CAD build for the part. Positions are in the model's coordinates, mm. Face numbers are marked on the shaded views. A direction names the side the tool comes from. Round coordinates to 2 decimals unless told otherwise and drop trailing zeros. Write each loop counter-clockwise with the first axis right and the second up, starting at its lowest first coordinate (ties: lowest second). Pieces come first, ordered by that corner, then holes. Notation, with made-up numbers: (23.5, 89.25) - (67.5, 89.25) arc R5 ccw to (67.5, 94.25) - close; hole circle Ø1 at (-30.75, 89.25). An arc over 180 degrees is marked (long way). Put each result on its own line as item: value. Start each with the question number.
Item 1: Pin check, flat tips, straight feed: pin 1 Ø1 at (y, z) = (18, 11) entering from -X; pin 2 Ø1.4 at (x, z) = (-10, 11) entering from +Y; pin 3 Ø0.8 at (x, y) = (8.5, 20.5) entering from +Z. Stop position of each tip, or through.
Item 2: Cut at A-A (y = 15). Give the cut face in (x, z), and give its area (3 significant figures).
Item 3: 3-axis set-ups, long thin cutter, end or side, ignore diameter. For the marked faces 1, 2, 3, 4 and 5: which of +Z, -Z, +X, -X, +Y, -Y reach the whole face in a straight line?
Item 4: Cut at B-B (x = -24). Give the cut face in (y, z).
Item 5: Drill centre lines: line 1 (Y direction, x = -3, z = 5.5); line 2 (X direction, y = -13, z = 1.75); line 3 (Y direction, x = 22, z = 13). Where is each one in solid material? Low to high. Write a range as from..to.
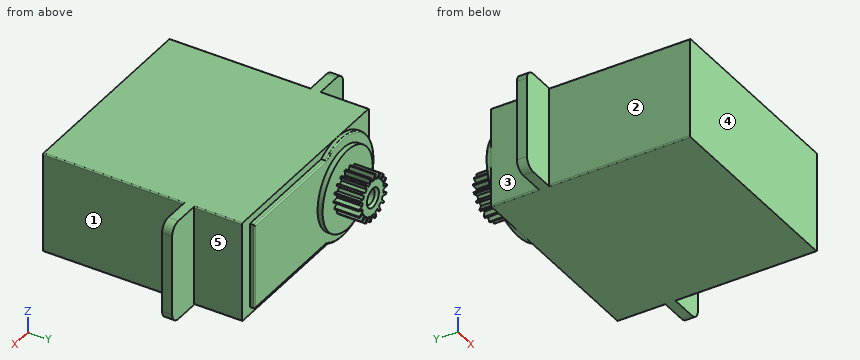
```python
from build123d import *

# Parameters (mm, degrees)
ESQUISSE1_W                  = 40.5
ESQUISSE1_H                  = 39.5
BOSS_EXTRU_1_DEPTH           = 20
ESQUISSE2_W                  = 20
ESQUISSE2_H                  = 2
BOSS_EXTRU_2_DEPTH           = 7
ESQUISSE3_W                  = 20
ESQUISSE3_H                  = 2
BOSS_EXTRU_3_DEPTH           = 7
CONG_1_R                     = 2
BOSS_EXTRU_4_DEPTH           = 1
ESQUISSE6_R                  = 8
BOSS_EXTRU_5_DEPTH           = 1
ESQUISSE7_R                  = 4.5
BOSS_EXTRU_6_DEPTH           = 5
ENL_V_START                  = -5
ENL_V_MAT_EXTRU_2_DEPTH      = 5
R_P_TITION_CIRCULAIRE2_COUNT = 18
ESQUISSE9_R                  = 1.4
ENL_V_MAT_EXTRU_3_DEPTH      = 5
CHANFREIN1_SIZE              = 0.5
CONG_3_R                     = 0.25
CONG_4_R                     = 0.25


with BuildPart() as part:
    # Esquisse1 → Boss.-Extru.1 (new body)
    with BuildSketch(Plane.XY):
        Rectangle(ESQUISSE1_W, ESQUISSE1_H)
    extrude(amount=BOSS_EXTRU_1_DEPTH)

    # Esquisse2 → Boss.-Extru.2 (add)
    with BuildSketch(Plane.ZY.offset(20.25)):
        with Locations((10, 9.25)):
            Rectangle(ESQUISSE2_W, ESQUISSE2_H)
    extrude(amount=BOSS_EXTRU_2_DEPTH)

    # Esquisse3 → Boss.-Extru.3 (add)
    with BuildSketch(Plane(origin=(20.25, 0, 0), x_dir=(0, 0, -1), z_dir=(1, 0, 0))):
        with Locations((-10, 9.25)):
            Rectangle(ESQUISSE3_W, ESQUISSE3_H)
    extrude(amount=BOSS_EXTRU_3_DEPTH)

    # Congé1
    cong_1_edges = [part.edges().sort_by_distance(p)[0] for p in [
        (-27.25, 9.25, 0),
        (-27.25, 9.25, 20),
        (27.25, 9.25, 20),
        (27.25, 9.25, 0),
    ]]
    fillet(cong_1_edges, radius=CONG_1_R)

    # Esquisse4 → Boss.-Extru.4 (add)
    with BuildSketch(Plane(origin=(0, 19.75, 0), x_dir=(1, 0, 0), z_dir=(0, 1, 0))):
        with BuildLine():
            Line((17.75, -1.5), (17.75, -18.5))
            Line((17.75, -18.5), (-5.001587186, -18.5))
            ThreePointArc((-5.001587186, -18.5), (-20.239786638, -10), (-5.001587186, -1.5))
            Line((-5.001587186, -1.5), (17.75, -1.5))
        make_face()
    extrude(amount=BOSS_EXTRU_4_DEPTH)

    # Esquisse6 → Boss.-Extru.5 (add)
    with BuildSketch(Plane(origin=(0, 20.75, 0), x_dir=(1, 0, 0), z_dir=(0, 1, 0))):
        with Locations(Location((-10.25, -10, 0), (0, 0, 270))):
            Circle(ESQUISSE6_R)
    extrude(amount=BOSS_EXTRU_5_DEPTH)

    # Esquisse7 → Boss.-Extru.6 (add)
    with BuildSketch(Plane(origin=(0, 21.75, 0), x_dir=(1, 0, 0), z_dir=(0, 1, 0))):
        with Locations(Location((-10.25, -10, 0), (0, 0, 270))):
            Circle(ESQUISSE7_R)
    extrude(amount=BOSS_EXTRU_6_DEPTH)

    # Esquisse8 → Enlèv. mat.-Extru.2 (cut)
    with BuildSketch(Plane(origin=(0, 26.75, 0), x_dir=(1, 0, 0), z_dir=(0, 1, 0)).offset(ENL_V_START)):
        with BuildLine():
            Line((-10.606352849, -6.656584169), (-10.903477232, -5.547700874))
            ThreePointArc((-10.903477232, -5.547700874), (-10.272597671, -5.50005674), (-9.641271425, -5.541362369))
            Line((-9.641271425, -5.541362369), (-9.940094206, -6.656584169))
            Line((-9.940094206, -6.656584169), (-10.606352849, -6.656584169))
        make_face()
    enl_v_mat_extru_2 = extrude(amount=ENL_V_MAT_EXTRU_2_DEPTH, mode=Mode.SUBTRACT)

    # Répétition circulaire2: Enlèv. mat.-Extru.2 ×18 about axis
    r_p_tition_circulaire2_axis = Axis((-10.249601616, 0, 10.07055578), (0, 1, 0))
    for i in range(1, R_P_TITION_CIRCULAIRE2_COUNT):
        add(enl_v_mat_extru_2.rotate(r_p_tition_circulaire2_axis, i * 360 / R_P_TITION_CIRCULAIRE2_COUNT), mode=Mode.SUBTRACT)

    # Esquisse9 → Enlèv. mat.-Extru.3 (cut)
    with BuildSketch(Plane(origin=(0, 26.75, 0), x_dir=(1, 0, 0), z_dir=(0, 1, 0))):
        with Locations(Location((-10.249601616, -10.07055578, 0), (0, 0, 270))):
            Circle(ESQUISSE9_R)
    extrude(amount=-ENL_V_MAT_EXTRU_3_DEPTH, mode=Mode.SUBTRACT)

    # Chanfrein1
    chanfrein1_edges = [part.edges().sort_by_distance(p)[0] for p in [
        (-10.249601616, 26.75, 8.67055578),
    ]]
    chamfer(chanfrein1_edges, length=CHANFREIN1_SIZE)

    # Congé3
    cong_3_edges = [part.edges().sort_by_distance(p)[0] for p in [
        (6.374206407, 20.75, 1.5),
        (-20.239786638, 20.75, 10),
        (6.374206407, 20.75, 18.5),
        (17.75, 20.75, 10),
    ]]
    fillet(cong_3_edges, radius=CONG_3_R)

    # Congé4
    cong_4_edges = [part.edges().sort_by_distance(p)[0] for p in [
        (-20.25, 15, 20),
        (-20.25, -5.75, 0),
        (-20.25, -5.75, 20),
        (20.25, 15, 0),
        (20.25, 15, 20),
        (20.25, -5.75, 20),
        (-20.25, 15, 0),
        (20.25, -5.75, 0),
    ]]
    fillet(cong_4_edges, radius=CONG_4_R)


solid = part.part
```
Output values:
1. pin 1: x = -20.25
1. pin 2: y = 26.51
1. pin 3: z = 18.5
2. outline: (-20.25, 0.25) arc R0.25 ccw to (-20, 0) - (20, 0) arc R0.25 ccw to (20.25, 0.25) - (20.25, 19.75) arc R0.25 ccw to (20, 20) - (-20, 20) arc R0.25 ccw to (-20.25, 19.75) - close
2. area: 810 mm2
3. face 1: +Z, -Z, +X, -Y
3. face 2: +Z, -Z, -X, -Y
3. face 3: +Z, -Z, -X, +Y
3. face 4: +Z, -Z, +X, -X, -Y
3. face 5: +Z, -Z, +X, +Y
4. outline: (8.25, 0) - (10.25, 0) - (10.25, 20) - (8.25, 20) - close
5. line 1: -19.75..20.75
5. line 2: -20.25..20.25
5. line 3: 8.25..10.25
